Source: CAD feature listing. Evaluate the final solid. Frame: model axes, mm. Face numbers are marked on the shaded views. A direction names the side the tool comes from. Round coordinates to 2 decimals unless told otherwise and drop trailing zeros. Order: outer loops, then holes, each group sorted by start corner. A loop starts at its lowest first (then second) coordinate and runs counter-clockwise, first axis right, second up. Notation, with made-up numbers: (23, -26) -> (36, -26) arc R23 cw to (36, -13) -> close; hole circle Ø1 at (22.5, 30). An arc over 180 degrees is marked (long way). Answer as CSV lines item,"result".
from build123d import *

# Parameters (mm, degrees)
F0_W     = 101.6
F0_H     = 101.6
F1_DEPTH = 31.75
F2_W     = 11.43
F2_H     = 3.175
F3_DEPTH = 27.94
F4_W     = 25.4
F4_H     = 12.7
F5_DEPTH = 17.272


with BuildPart() as f1:
    # F0 (on Top) → F1 (new body, symmetric)
    with BuildSketch(Plane.XY):
        Rectangle(F0_W, F0_H)
    extrude(amount=F1_DEPTH, both=True)

    # F2 (on face) → F3 (cut)
    with BuildSketch(Plane(origin=(0, 0, -31.75), x_dir=(1, 0, 0), z_dir=(0, 0, -1))):
        Polygon((12.7, 0), (0, 0), (-27.94, 0), (-27.94, -10.16), (12.7, -10.16), (12.7, -3.175), align=None)
        Polygon((-27.94, 0), (0, 0), (12.7, 0), (12.7, 3.175), (12.7, 10.16), (-27.94, 10.16), align=None)
        with Locations((18.415, 1.5875)):
            Rectangle(F2_W, F2_H)
        with Locations((18.415, -1.5875)):
            Rectangle(F2_W, F2_H)
    extrude(amount=-F3_DEPTH, mode=Mode.SUBTRACT)

    # F4 (on face) → F5 (cut)
    with BuildSketch(Plane.XZ.offset(50.8)):
        Polygon((-38.1, 0), (-25.4, 0), (-25.4, 25.4), (-25.4, 31.75), (-38.1, 31.75), align=None)
        Polygon((-25.4, 0), (0, 0), (0, 31.75), (-19.05, 31.75), (-19.05, 25.4), (-25.4, 25.4), align=None)
        Polygon((0, 31.75), (0, 0), (25.4, 0), (25.4, 25.4), (19.05, 25.4), (19.05, 31.75), align=None)
        with Locations((12.7, -6.35)):
            Rectangle(F4_W, F4_H)
        Polygon((0, -12.7), (0, 0), (-25.4, 0), (-25.4, -1.27), (-19.05, -1.27), (-19.05, -7.62), (-25.4, -7.62), (-25.4, -12.7), align=None)
    extrude(amount=-F5_DEPTH, mode=Mode.SUBTRACT)


solid = f1.part
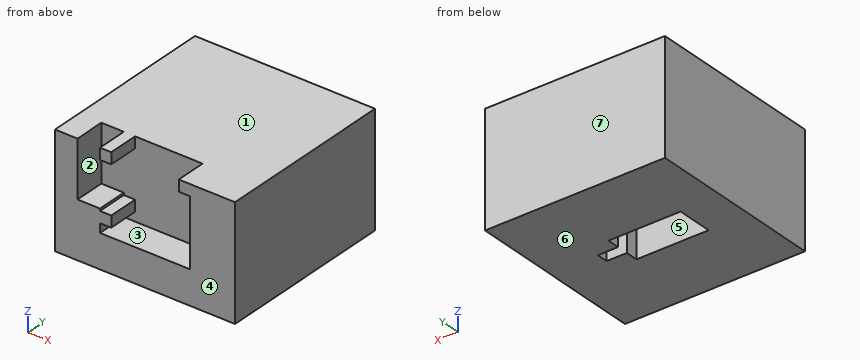
1. Section query C-C on y = -1. Return loops of the section in (x, z), and give its area (3 significant figures).
Results below:
outline,"(-50.8, -31.75) -> (-27.94, -31.75) -> (-27.94, -3.81) -> (24.13, -3.81) -> (24.13, -31.75) -> (50.8, -31.75) -> (50.8, 31.75) -> (-50.8, 31.75) -> close"
area,"5,000 mm2"
2. Section query A-A on z = -26.5. Return loops of the section in (x, y) (3 decimals), and give its area (3 significant figures).
Results below:
outline,"(-50.8, -50.8) -> (50.8, -50.8) -> (50.8, 50.8) -> (-50.8, 50.8) -> close; hole (-27.94, -10.16) -> (12.7, -10.16) -> (12.7, -3.175) -> (24.13, -3.175) -> (24.13, 3.175) -> (12.7, 3.175) -> (12.7, 10.16) -> (-27.94, 10.16) -> close"
area,"9,420 mm2"
3. Reachability of the marked faces 1, 2 and 3 from +Z, -Z, +X, -X, +Y, -Y: full face, straight path, thin tool, end or side. Return the list, or none.
Results below:
face 1,"+Z, +X, -X, +Y, -Y"
face 2,"+Z, -Y"
face 3,"-Y"
4. Section query D-D on z = 22.5. Return loops of the section in (x, y), and give its area (3 significant figures).
Results below:
outline,"(-50.8, -50.8) -> (-38.1, -50.8) -> (-38.1, -33.53) -> (25.4, -33.53) -> (25.4, -50.8) -> (50.8, -50.8) -> (50.8, 50.8) -> (-50.8, 50.8) -> close"
area,"9,230 mm2"
5. Mould query, pull axis Y, two halves, no side actions, for the marked faces 4, 5, 6 and 7. Classes: released by +Y, released by -Y, zero draft, split by the parting line, or undercut.
Results below:
face 4,"released by -Y"
face 5,"undercut"
face 6,"zero draft"
face 7,"released by +Y"
6. Section query B-B on x = 16.5. Return loops of the section in (y, z) (3 decimals).
Results below:
outline,"(-50.8, -31.75) -> (-3.175, -31.75) -> (-3.175, -3.81) -> (3.175, -3.81) -> (3.175, -31.75) -> (50.8, -31.75) -> (50.8, 31.75) -> (-33.528, 31.75) -> (-33.528, -12.7) -> (-50.8, -12.7) -> close"
7. Line query: L1, parallel to Y at x = -20.5, z = -21; L2, parallel to Y at x = -22, z = 1; L3, parallel to X at y = -42.5, z = 23. Output: solid intervals per line, ascending. Write a range as [from, to].
Results below:
L1,"[-50.8, -10.16], [10.16, 50.8]"
L2,"[-33.53, 50.8]"
L3,"[-50.8, -38.1], [25.4, 50.8]"
8. Pin query (flat end, axial travel): pin 1 (4 mm diameter, centred on x = -17, z = 18, fed in from -Y); pin 2 (14 mm diameter, centred on x = -33, y = -42.5, fed in from +Z); pin 3 (5 mm diameter, centred on x = -12, y = -44.5, fed in from +Z). Return the tip coordinate at first contact, or that it passes through.
Results below:
pin 1,"y = -33.53"
pin 2,"z = 31.75"
pin 3,"z = -12.7"
